For this review, take the finished solid that the model builds, in its own axes (mm). A direction names the side the tool comes from. Coordinates: 2 decimals unless noted, no trailing zeros. Loops run counter-clockwise (first coordinate to the right, second up) from the corner with the lowest first, then second, coordinate; pieces in that order, holes last. Notation, with made-up numbers: (-28, 56) -> (22, 56) arc R9 cw to (22, 64) -> close; hole circle Ø5 at (75, 12). An arc over 180 degrees is marked (long way). Use a Markdown table: item, result.
from build123d import *

# Parameters (mm, degrees)
F0_W        = 100
F0_H        = 70
F1_DEPTH    = 100
F2_T        = -12.7
F3_T1_DEPTH = 290.5
F4_T1_DEPTH = 290.5
F5_W        = 9
F5_H        = 32
F6_DEPTH    = 50.8
F7_W        = 9
F7_H        = 30
F8_DEPTH    = 50.8
F9_W        = 10
F9_H        = 10
F10_DEPTH   = 83.82


# Not quite as in the source:
# - a fillet or chamfer that OpenCascade refuses, or shapes differently, is made with other operations: its cross-section is extruded or revolved along the edge and cut away or added


with BuildPart() as f1:
    # F0 (on Front) → F1 (new body)
    with BuildSketch(Plane.XZ):
        with Locations((-15.9141167998, -52.9208671927)):
            Rectangle(F0_W, F0_H)
    extrude(amount=F1_DEPTH)

    # F2
    f2_openings = [f1.faces().sort_by_distance(p)[0] for p in [
        (-15.914117, -50, -87.920867),
    ]]
    offset(amount=F2_T, openings=f2_openings)

    # F3: fillet of radius 38.1 on 1 edges, made by hand

    # F3_s2 → F3_t1 (cut)
    with BuildSketch(Plane.XZ.offset(-95.25)):
        with BuildLine():
            add(Edge.make_bspline(
                [(34.0858832002, -56.0208671927), (34.0858832002, -17.9208671927), (-4.0141167998, -17.9208671927)],
                knots=[0, 0, 0, 1, 1, 1], degree=2, weights=[1, 1, 1]))
            Line((-4.0141167998, -17.9208671927), (34.0858832002, -17.9208671927))
            Line((34.0858832002, -17.9208671927), (34.0858832002, -56.0208671927))
        make_face()
    extrude(amount=F3_T1_DEPTH, mode=Mode.SUBTRACT)

    # F4: fillet of radius 38.1 on 1 edges, made by hand

    # F4_s2 → F4_t1 (cut)
    with BuildSketch(Plane.XZ.offset(-95.25)):
        with BuildLine():
            add(Edge.make_bspline(
                [(-27.8141167998, -17.9208671927), (-65.9141167998, -17.9208671927), (-65.9141167998, -56.0208671927)],
                knots=[0, 0, 0, 1, 1, 1], degree=2, weights=[1, 1, 1]))
            Line((-65.9141167998, -56.0208671927), (-65.9141167998, -17.9208671927))
            Line((-65.9141167998, -17.9208671927), (-27.8141167998, -17.9208671927))
        make_face()
    extrude(amount=F4_T1_DEPTH, mode=Mode.SUBTRACT)

    # F5 (on face) → F6 (cut)
    with BuildSketch(Plane(origin=(-65.9141167998, 0, 0), x_dir=(0, -1, 0), z_dir=(-1, 0, 0))):
        with Locations((18.5, -22.9208671927)):
            Rectangle(F5_W, F5_H)
    extrude(amount=-F6_DEPTH, mode=Mode.SUBTRACT)

    # F7 (on face) → F8 (cut)
    with BuildSketch(Plane.YZ.offset(34.0858832002)):
        with Locations((-81.5, -23.9208671927)):
            Rectangle(F7_W, F7_H)
    extrude(amount=-F8_DEPTH, mode=Mode.SUBTRACT)

    # F9 (on face) → F10 (join)
    with BuildSketch(Plane(origin=(21.3858832002, 0, 0), x_dir=(0, -1, 0), z_dir=(-1, 0, 0))):
        with Locations((25, -46.9208671927)):
            Rectangle(F9_W, F9_H)
        with Locations((75, -46.9208671927)):
            Rectangle(F9_W, F9_H)
    extrude(amount=F10_DEPTH)


solid = f1.part
(1) Take a section at C-C on x = 19.5. State how many separate pieces and enclosed holes the cut face has, plus the area to 3 significant figures.
Found:
| item | result |
|---|---|
| separate pieces | 4 |
| enclosed holes | 0 |
| area | 2,310 mm^2 |
(2) Take a section at B-B on z = -78.5. Write out the cut boundary in (x, y).
Found:
| item | result |
|---|---|
| outline | (-65.91, -100) -> (34.09, -100) -> (34.09, 0) -> (-65.91, 0) -> close; hole (-53.21, -87.3) -> (21.39, -87.3) -> (21.39, -12.7) -> (-53.21, -12.7) -> close |
(3) Take a section at A-A on x = -9.5. Write out the cut boundary in (y, z), plus the area to 3 significant figures.
Found:
| item | result |
|---|---|
| outline | (-100, -87.92) -> (-87.3, -87.92) -> (-87.3, -30.62) -> (-86, -30.62) -> (-86, -17.92) -> (-100, -17.92) -> close; (-80, -51.92) -> (-70, -51.92) -> (-70, -41.92) -> (-80, -41.92) -> close; (-77, -30.62) -> (-12.7, -30.62) -> (-12.7, -87.92) -> (0, -87.92) -> (0, -17.92) -> (-77, -17.92) -> close; (-30, -51.92) -> (-20, -51.92) -> (-20, -41.92) -> (-30, -41.92) -> close |
| area | 2,810 mm^2 |
(4) For faces 5 (the face through (-15, -25, -41.921)), 6 (the face through (8, -86, -26)), 7 (the face through (-16, -87.3, -59)), list the 3-axis set-ups (+Z, -Z, +X, -X, +Y, -Y) from which the entire face can be reached by the end or side of a thin tool; tool diameter is ignored.
Found:
| item | result |
|---|---|
| face 5 | none |
| face 6 | +Z, +X |
| face 7 | -Z |
(5) For line 1 along Y through (x, z) = (-35, -45.5); line 2 along X through (y, z) = (-28, -84); line 3 along Y through (x, z) = (20.5, -84), list the stretches that pass through material, from the lowest coordinate up.
Found:
| item | result |
|---|---|
| line 1 | y = -100 to -87.3, -80 to -70, -30 to -20, -12.7 to 0 |
| line 2 | x = -65.91 to -53.21, 21.39 to 34.09 |
| line 3 | y = -100 to -87.3, -12.7 to 0 |
(6) Mouldability with a two-part tool opening along Y and no side actions: class faces 1 (the face through (34.086, -49, -72)), 2 (the face through (-40, -14, -26)), 3 (the face through (-17, 0, -52)), 4 (the face through (-15, -25, -51.921)) as pulls with the +Y half, pulls with the -Y half, needs draft (parallel to the pull), parting line crosses it, or undercut.
Found:
| item | result |
|---|---|
| face 1 | needs draft |
| face 2 | undercut |
| face 3 | pulls with the +Y half |
| face 4 | undercut |
(7) For pin 1 Ø7 at (y, z) = (-79.5, -27) entering from +X; pin 2 Ø4.5 at (x, y) = (24.5, -83) entering from +Z; pin 3 Ø10 at (y, z) = (-19.5, -21) entering from -X, all flat-tipped, find the tip position at first contact; note any pin that passes through.
Found:
| item | result |
|---|---|
| pin 1 | stops at x = 26.37 |
| pin 2 | stops at z = -38.92 |
| pin 3 | stops at x = -53 |
